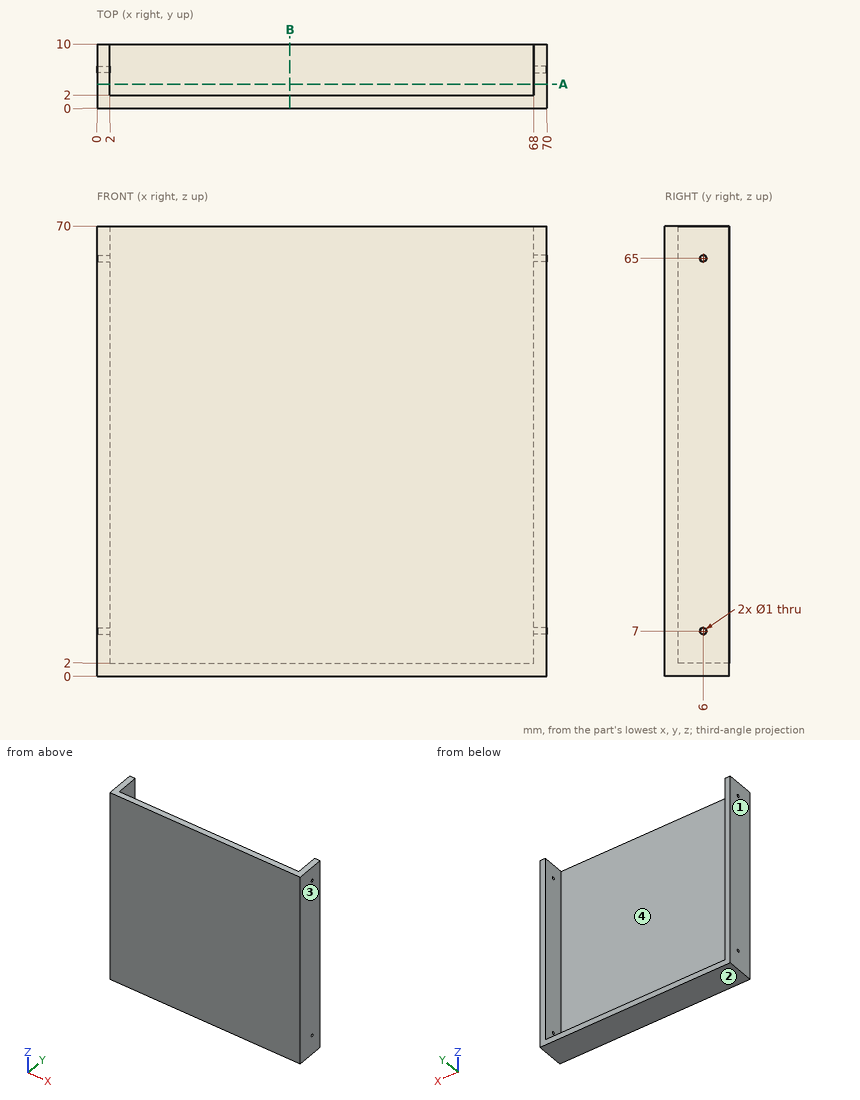
Print and shaded views of the part. All mm, measured from the part's lowest x, y and z. Round coordinates to 2 decimals unless told otherwise and drop trailing zeros. Order: outer loops, then holes, each group sorted by start corner. A loop starts at its lowest first (then second) coordinate and runs counter-clockwise, first axis right, second up.
Q1. Two-plate mould, pull along X, no slides. Class the marked faces 1, 2, 3 and 4: pulls with the +X half, pulls with the -X half, needs draft (parallel to the pull), parting line crosses it, or undercut.
Q2. Slice it at A-A (y = 3.75). Write the cut outline in (x, z).
Q3. Drop flat-ended pins along their axis: pin 1 (3 mm diameter, centred on x = 37, z = 13.5, fed in from +Y); pin 2 (2.5 mm diameter, centred on x = 21, y = 4, fed in from +Z). Give the stop position or say it passes through.
Q4. Slice it at B-B (x = 30). Write the cut outline in (y, z).
Q5. Wall check: L1, parallel to Z at x = 69, y = 6; L2, parallel to X at y = 5, z = 40; L3, parallel to Y at x = 69, z = 7. Give the ranges that are in metal, low to high.
Results below:
1. face 1: pulls with the -X half
1. face 2: needs draft
1. face 3: pulls with the +X half
1. face 4: undercut
2. outline: (0, 0) - (70, 0) - (70, 70) - (68, 70) - (68, 2) - (2, 2) - (2, 70) - (0, 70) - close
3. pin 1: stops at y = 2
3. pin 2: stops at z = 2
4. outline: (0, 0) - (10, 0) - (10, 2) - (2, 2) - (2, 70) - (0, 70) - close
5. L1: z = 0 to 6.5, 7.5 to 64.5, 65.5 to 70
5. L2: x = 0 to 2, 68 to 70
5. L3: y = 0 to 5.5, 6.5 to 10
